```python
from build123d import *

# Parameters (mm, degrees)
SKETCH1_W           = 161.724310644
SKETCH1_H           = 96.872862076
BOSS_EXTRUDE1_DEPTH = 50.8
SKETCH2_R           = 20.831004362
CUT_EXTRUDE1_DEPTH  = 51.8
SKETCH3_RX          = 14.294101548
SKETCH3_RY          = 7.07473185
BOSS_EXTRUDE2_DEPTH = 76.2


with BuildPart() as part:
    # Sketch1 → Boss-Extrude1 (new body)
    with BuildSketch(Plane.XY):
        Rectangle(SKETCH1_W, SKETCH1_H)
    extrude(amount=BOSS_EXTRUDE1_DEPTH)

    # Sketch2 → Cut-Extrude1 (cut, through all)
    with BuildSketch(Plane.XY.offset(50.8)):
        with Locations((-5.525694513, 15.560482637)):
            Circle(SKETCH2_R)
    extrude(amount=-CUT_EXTRUDE1_DEPTH, mode=Mode.SUBTRACT)

    # Sketch3 → Boss-Extrude2 (add)
    with BuildSketch(Plane(origin=(80.862155322, 0, 0), x_dir=(0, 0, -1), z_dir=(1, 0, 0))):
        with Locations(Location((-22.034477626, 0), (0, 0, -90))):
            Ellipse(SKETCH3_RX, SKETCH3_RY)
    extrude(amount=BOSS_EXTRUDE2_DEPTH)


solid = part.part
```
Part model, mm, in its own coordinate system. Round coordinates to 2 decimals unless told otherwise and drop trailing zeros. Loops run counter-clockwise (first coordinate to the right, second up) from the corner with the lowest first, then second, coordinate; pieces in that order, holes last.
Item 1: Drop flat-ended pins along their axis: P1, Ø1.5, axis at y = 1, z = 36, coming from the +X side; P2, Ø4, axis at x = 13, y = 15.5, coming from the +Z side; P3, Ø1, axis at x = 109.5, y = -10, coming from the +Z side. Give the stop position or say it passes through.
Item 2: Drill centre lines: line 1 (X direction, y = 41.5, z = 46); line 2 (X direction, y = 24, z = 2.5); line 3 (X direction, y = 25, z = 32.5). Where is each one in solid material? Low to high.
Item 3: Mould opens along Y. For faces 1 (the face through (-1, -48.436, 25)), 2 (the face through (-1, -10, 50.8)), 3 (the face through (14.343, 21.818, 25.756)), 4 (the face through (-1, 48.436, 25)) say: +Y half, -Y half, draft (parallel to the pull), parting line (faces both ways), or undercut.
Item 4: Cut at C-C, the plane y = -17.5. Give the cut face in (x, z), then the cut area to 3 significant figures.
Item 5: Cut at A-A, the plane x = -11. Give the cut face in (y, z).
Item 6: Cut at B-B, the plane z = 39. Give the cut face in (x, y).
A:
1. P1: stops at x = 80.86
1. P2: passes through
1. P3: stops at z = 27.32
2. line 1: x = -80.86 to 80.86
2. line 2: x = -80.86 to -24.57, 13.52 to 80.86
2. line 3: x = -80.86 to -24.1, 13.04 to 80.86
3. face 1: -Y half
3. face 2: draft
3. face 3: undercut
3. face 4: +Y half
4. outline: (-80.86, 0) - (80.86, 0) - (80.86, 50.8) - (-80.86, 50.8) - close
4. area: 8,220 mm2
5. outline: (-48.44, 0) - (-4.54, 0) - (-4.54, 50.8) - (-48.44, 50.8) - close; (35.66, 0) - (48.44, 0) - (48.44, 50.8) - (35.66, 50.8) - close
6. outline: (-80.86, -48.44) - (80.86, -48.44) - (80.86, 48.44) - (-80.86, 48.44) - close; hole circle Ø41.66 at (-5.53, 15.56)
